For this review, take the finished solid that the model builds, in its own axes (mm). A direction names the side the tool comes from. Coordinates: 2 decimals unless noted, no trailing zeros. Order: outer loops, then holes, each group sorted by start corner. A loop starts at its lowest first (then second) coordinate and runs counter-clockwise, first axis right, second up. Notation, with made-up numbers: (61.5, -1) - (96.5, -1) arc R29 ccw to (96.5, 27) - close; hole circle Ø7 at (35.25, 3). An arc over 180 degrees is marked (long way). One line per item, written item: value. Start each with the question number.
(1) For faces 5 (the flat face through (38, -34, 10)), 6 (the flat face through (6, -38, 10)), 7 (the flat face through (35, -32.5, 10)), list the 3-axis set-ups (+Z, -Z, +X, -X, +Y, -Y) from which the entire face can be reached by the end or side of a thin tool; tool diameter is ignored.
(2) Consider section B-B on z = 9. Write out the cut boundary in (x, y).
(3) To check wall thickness, follow line 1 along X through (y, z) = (-20, -1); line 2 along Y through (x, z) = (5.5, 14); line 3 along Y through (x, z) = (20, -1.25). State the ranges of each line that lie inside material, in increasing order.
(4) Consider section A-A on y = -20. Write out the cut boundary in (x, z).
(5) Consider section D-D on y = -12. Write out the cut boundary in (x, z).
(6) Mouldability with a two-part tool opening along X and no side actions: class faces 1 (the flat face through (7.5, -35, 10)), 2 (the flat face through (18, -20, -3)), 3 (the flat face through (38, -6, 10)), 4 (the flat face through (17.6, -20.1, -10)) as released by +X, released by -X, zero draft, split by the parting line, or undercut.
(7) Clearance check with flat-ended pins moving along their axes: pin 1 (1 mm diameter, centred on y = -34, z = 8, fed in from +X); pin 2 (2 mm diameter, centred on y = -25.5, z = 7.5, fed in from +X); pin 3 (4.5 mm diameter, centred on y = -5.5, z = 12.5, fed in from -X); pin 4 (3 mm diameter, centred on x = 23.5, y = -29.5, fed in from +Z). State where each tip first meets the part, or that it passes through.
(8) Consider section C-C on x = 20. Write out the cut boundary in (y, z).
```python
from build123d import *

# Parameters (mm, degrees)
EXTRUDE002_DEPTH = 20
SKETCH003_R      = 10
EXTRUDE_DEPTH    = 10
SKETCH_W         = 40
SKETCH_H         = 40
PAD_DEPTH        = 5
PAD001_DEPTH     = 10


with BuildPart() as extrude002:
    # Sketch008 (on Face1 of CopyExtrude) → Extrude002 (new body)
    with BuildSketch(Plane(origin=(0, 0, -10), x_dir=(1, 0, 0), z_dir=(0, 0, -1))):
        with BuildLine():
            ThreePointArc((18, 16.535898), (24, 20), (18, 23.464102))
            Line((18, 23.464102), (18, 16.535898))
        make_face()
    extrude(amount=-EXTRUDE002_DEPTH)


with BuildPart() as valec:
    # Sketch003 → Extrude (new body)
    with BuildSketch(Plane(origin=(0, 0, 0), x_dir=(1, 0, 0), z_dir=(0, 0, -1))):
        with Locations((20, 20)):
            Circle(SKETCH003_R)
    extrude(amount=EXTRUDE_DEPTH)


with BuildPart() as obj1:
    # Sketch → Pad (new body)
    with BuildSketch(Plane.XY):
        with Locations((20, -20)):
            Rectangle(SKETCH_W, SKETCH_H)
    extrude(amount=PAD_DEPTH)

    # Sketch001 (on Face6 of Pad) → Pad001 (join)
    with BuildSketch(Plane.XY.offset(5)):
        with BuildLine():
            Line((4, -2), (7.5, -2))
            Line((7.5, -2), (7.5, -7.5))
            Line((7.5, -7.5), (2, -7.5))
            Line((2, -7.5), (2, -4))
            ThreePointArc((4, -2), (2.585786, -2.585786), (2, -4))
        make_face()
        with BuildLine():
            Line((38, -7.5), (38, -4))
            ThreePointArc((38, -4), (37.414214, -2.585786), (36, -2))
            Line((36, -2), (32.5, -2))
            Line((32.5, -2), (32.5, -7.5))
            Line((32.5, -7.5), (38, -7.5))
        make_face()
        with BuildLine():
            Line((7.5, -32.5), (2, -32.5))
            Line((2, -32.5), (2, -36))
            ThreePointArc((2, -36), (2.585786, -37.414214), (4, -38))
            Line((4, -38), (7.5, -38))
            Line((7.5, -38), (7.5, -32.5))
        make_face()
        with BuildLine():
            Line((32.5, -38), (32.5, -32.5))
            Line((32.5, -32.5), (38, -32.5))
            Line((38, -32.5), (38, -36))
            ThreePointArc((36, -38), (37.414214, -37.414214), (38, -36))
            Line((36, -38), (32.5, -38))
        make_face()
    extrude(amount=PAD001_DEPTH)

    # Fusion: union Valec
    add(valec.part)

    # Cut: cut Extrude002
    add(extrude002.part, mode=Mode.SUBTRACT)


solid = obj1.part
```
Geometry check:
1. face 5: +Z, +X, +Y, -Y
1. face 6: +Z, +X, -X, -Y
1. face 7: +Z, +X, -X
2. outline: (2, -36) arc R2 ccw to (4, -38) - (7.5, -38) - (7.5, -32.5) - (2, -32.5) - close; (2, -7.5) - (7.5, -7.5) - (7.5, -2) - (4, -2) arc R2 ccw to (2, -4) - close; (32.5, -38) - (36, -38) arc R2 ccw to (38, -36) - (38, -32.5) - (32.5, -32.5) - close; (32.5, -7.5) - (38, -7.5) - (38, -4) arc R2 ccw to (36, -2) - (32.5, -2) - close
3. line 1: x = 10 to 18, 24 to 30
3. line 2: y = -38 to -32.5, -7.5 to -2
3. line 3: y = -30 to -24, -16 to -10
4. outline: (0, 0) - (10, 0) - (10, -10) - (18, -10) - (18, 5) - (0, 5) - close; (24, -10) - (30, -10) - (30, 0) - (40, 0) - (40, 5) - (24, 5) - close
5. outline: (0, 0) - (14, 0) - (14, -10) - (26, -10) - (26, 0) - (40, 0) - (40, 5) - (0, 5) - close
6. face 1: undercut
6. face 2: undercut
6. face 3: released by +X
6. face 4: zero draft
7. pin 1: stops at x = 38
7. pin 2: passes through
7. pin 3: stops at x = 2
7. pin 4: stops at z = 5
8. outline: (-40, 0) - (-30, 0) - (-30, -10) - (-24, -10) - (-24, 5) - (-40, 5) - close; (-16, -10) - (-10, -10) - (-10, 0) - (0, 0) - (0, 5) - (-16, 5) - close
